Design review of the part built by this model. Coordinates are the model's own, in mm. Round coordinates to 2 decimals unless told otherwise and drop trailing zeros. Loops run counter-clockwise (first coordinate to the right, second up) from the corner with the lowest first, then second, coordinate; pieces in that order, holes last. Notation, with made-up numbers: M 9.5,40.5 L 31.5,40.5 A20 cw 31.5,75.5 Z; hole C -38.5,-13.5 d6. An arc over 180 degrees is marked long. One line per item, written item: value. Start each with the question number.
Item 1: We need section A-A (z = -58.5). Write out the cut boundary in (x, y).
Item 2: We need section C-C (z = 76). Write out the cut boundary in (x, y), then the cut area to 3 significant figures.
Item 3: Clearance check with flat-ended pins moving along their axes: pin 1 (4.5 mm diameter, centred on y = 80.01, z = 12.7, fed in from +X); pin 2 (12 mm diameter, centred on x = -0.5, z = -43.5, fed in from +Y); pin 3 (3 mm diameter, centred on y = 80.01, z = 38.1, fed in from -X); pin 4 (1.9 mm diameter, centred on x = -26.5, y = 2, fed in from -Z). State where each tip first meets the part, or that it passes through.
Item 4: Mouldability with a two-part tool opening along X and no side actions: class faces 1 (the flat face through (59.69, 52, -1)), 2 (the flat face through (-63.5, 50, -1)), 3 (the flat face through (-1, 3.81, 31)), 4 (the cylindrical face through (-61.62, 9.17, -92.91)) as released by +X, released by -X, zero draft, split by the parting line, or undercut.
Item 5: For line 1 along Z through (x, y) = (-61.3, 80.01); line 2 along Z through (x, y) = (61.8, 55.45); line 3 along X through (y, z) = (18, 46), list the stretches that pass through material, from the lowest coordinate up.
Item 6: We need section B-B (y = 73). Write out the cut boundary in (x, z).
Item 7: We need section D-D (x = 5). Write out the cut boundary in (y, z).
Autodesk Inventor part; units mm, degrees
ref_plane "YZ Plane" through (0, 0, 0) normal (1, 0, 0) x (0, 1, 0)
ref_plane "XZ Plane" through (0, 0, 0) normal (0, 1, 0) x (-1, 0, 0)
ref_plane "XY Plane" through (0, 0, 0) normal (0, 0, 1) x (1, 0, 0)
sketch "Sketch1" plane through (0, 0, 0) normal (0, 1, 0) x (-1, 0, 0)
  line L0 (-63.5, -101.6) -> (63.5, -101.6)
  line L1 (63.5, -101.6) -> (63.5, 101.6)
  line L2 (63.5, 101.6) -> (-63.5, 101.6)
  line L3 (-63.5, 101.6) -> (-63.5, -101.6)
  line L4 (-63.5, -101.6) -> (63.5, 101.6) construction
  line L5 (63.5, -101.6) -> (-63.5, 101.6) construction
  point P0 (0, 0)
  dimension "d0" = 127
  dimension "d1" = 203.2
extrude "Extrusion1" add sketch "Sketch1" along normal blind 101.6
sketch "Sketch3" plane through (0, 101.6, 0) normal (0, 1, 0) x (1, 0, 0)
  line L0 (63.5, 101.6) -> (-63.5, 101.6)
  line L1 (59.69, -101.6) -> (-59.69, -101.6)
  line L2 (-59.69, -101.6) -> (-59.69, 101.6)
  line L3 (-59.69, 101.6) -> (59.69, 101.6)
  line L4 (59.69, 101.6) -> (59.69, -101.6)
  line L5 (59.69, -101.6) -> (-59.69, 101.6) construction
  line L6 (-59.69, -101.6) -> (59.69, 101.6) construction
  point P0 (0, 0)
  dimension "d4" = 119.38
extrude "Extrusion2" cut sketch "Sketch3" against normal blind 97.79
sketch "Sketch4" plane through (0, 3.81, 0) normal (0, 1, 0) x (1, 0, 0)
  line L0 (59.69, 101.6) -> (59.69, -101.6)
  line L1 (-59.69, 101.6) -> (59.69, 101.6)
  line L2 (59.69, 101.6) -> (-59.69, 101.6)
  line L3 (-59.69, 101.6) -> (-59.69, 38.1)
  line L4 (-59.69, 38.1) -> (59.69, 38.1)
  line L5 (59.69, 38.1) -> (59.69, 101.6)
  point P0 (0, 0)
  dimension "d7" = 63.5
extrude "Extrusion3" cut sketch "Sketch4" against normal blind 3.81
fillet "Fillet1" radius 30.48 2 edges at (61.595, 0, -101.6) (-61.595, 0, -101.6)
sketch "Sketch7" plane through (63.5, 0, 101.6) normal (1, 0, 0) x (0, 0, -1)
  circle A0 centre (189.7, 55.45) radius 1.85
  circle A1 centre (197.7, 47.45) radius 1.85
  circle A2 centre (181.7, 47.45) radius 1.85
  circle A3 centre (189.7, 39.45) radius 1.85
  point P0 (101.6, 0)
hole "Hole2" at (63.5, 55.45, -88.1) at (63.5, 47.45, -96.1) at (63.5, 47.45, -80.1) at (63.5, 39.45, -88.1) direction (-1, 0, 0) diameter 3.7 end through all
sketch "Sketch8" plane through (63.5, 0, 101.6) normal (1, 0, 0) x (0, 0, -1)
  circle A0 centre (63.5, 80.01) radius 1.85
  circle A1 centre (88.9, 80.01) radius 1.85
  point P0 (101.6, 0)
hole "Hole3" at (63.5, 80.01, 38.1) at (63.5, 80.01, 12.7) direction (-1, 0, 0) diameter 3.7 end through all
properties part number "Base Bucket"
A:
1. outline: M -63.5,0 L -59.69,0 L -59.69,101.6 L -63.5,101.6 Z; M 59.69,0 L 63.5,0 L 63.5,101.6 L 59.69,101.6 Z
2. outline: M -63.5,0 L 63.5,0 L 63.5,101.6 L 59.69,101.6 L 59.69,3.81 L -59.69,3.81 L -59.69,101.6 L -63.5,101.6 Z
2. area: 1,230 mm2
3. pin 1: x = 63.5
3. pin 2: y = 3.81
3. pin 3: through
3. pin 4: z = -38.1
4. face 1: undercut
4. face 2: released by -X
4. face 3: undercut
4. face 4: zero draft
5. line 1: -101.6 to 10.85, 14.55 to 36.25, 39.95 to 101.6
5. line 2: -101.6 to -89.95, -86.25 to 101.6
5. line 3: -63.5 to -59.69, 59.69 to 63.5
6. outline: M -63.5,-101.6 L -59.69,-101.6 L -59.69,101.6 L -63.5,101.6 Z; M 59.69,-101.6 L 63.5,-101.6 L 63.5,101.6 L 59.69,101.6 Z
7. outline: M 0,-38.1 L 3.81,-38.1 L 3.81,101.6 L 0,101.6 Z
